For this review, use the dimensioned drawing (mm, ordinates from the lowest corner) and the shaded views. A direction names the side the tool comes from. Coordinates: 2 decimals unless noted, no trailing zeros. Loops run counter-clockwise (first coordinate to the right, second up) from the corner with the lowest first, then second, coordinate; pieces in that order, holes last. Notation, with made-up numbers: M -22.75,27.5 L 34.25,27.5 A23 cw 34.25,47.5 Z; hole C -10.5,-32 d10. An arc over 180 degrees is marked long. One line per item, written item: value.
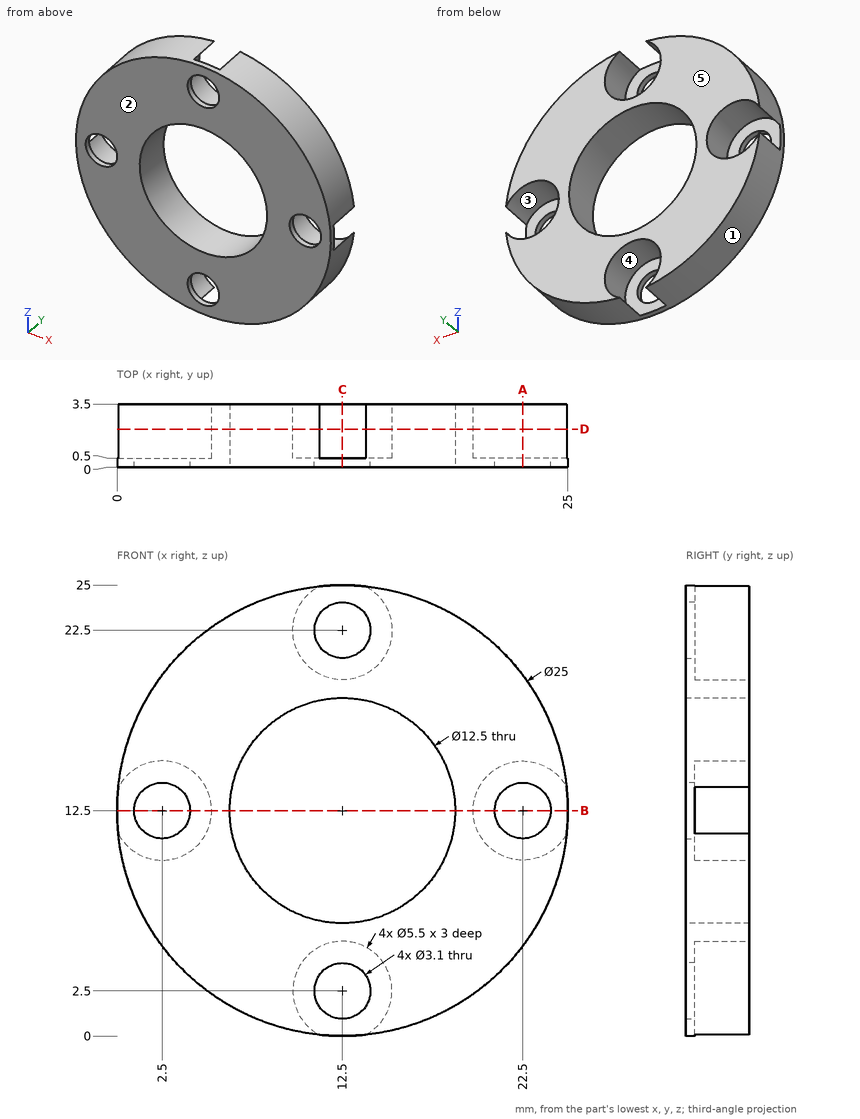
(1) Tool access review of the marked faces 4 and 5: name each direction out of +Z, -Z, +X, -X, +Y, -Y from which nothing blocks a thin tool from reaching the whole face with its end or side.
Reply:
face 4: +Y
face 5: +Z, -Z, +X, -X, +Y
(2) Mouldability with a two-part tool opening along Z and no side actions: class the marked faces 1, 2 and 3 as released by +Z, released by -Z, zero draft, split by the parting line, or undercut.
Reply:
face 1: split by the parting line
face 2: zero draft
face 3: undercut
(3) We need section C-C on x = 12.5. State the section outline as (y, z) points.
Reply:
outline: M 0,0 L 0.5,0 L 0.5,0.95 L 0,0.95 Z; M 0,4.05 L 0.5,4.05 L 0.5,5.25 L 3.5,5.25 L 3.5,6.25 L 0,6.25 Z; M 0,18.75 L 3.5,18.75 L 3.5,19.75 L 0.5,19.75 L 0.5,20.95 L 0,20.95 Z; M 0,24.05 L 0.5,24.05 L 0.5,25 L 0,25 Z
(4) We need section B-B on z = 12.5. State the section outline as (x, y) points.
Reply:
outline: M 0,0 L 0.95,0 L 0.95,0.5 L 0,0.5 Z; M 4.05,0 L 6.25,0 L 6.25,3.5 L 5.25,3.5 L 5.25,0.5 L 4.05,0.5 Z; M 18.75,0 L 20.95,0 L 20.95,0.5 L 19.75,0.5 L 19.75,3.5 L 18.75,3.5 Z; M 24.05,0 L 25,0 L 25,0.5 L 24.05,0.5 Z
(5) We need section A-A on x = 22.5. State the section outline as (y, z) points, then the cut area to 4 significant figures.
Reply:
outline: M 0,5 L 3.5,5 L 3.5,9.75 L 0.5,9.75 L 0.5,10.95 L 0,10.95 Z; M 0,14.05 L 0.5,14.05 L 0.5,15.25 L 3.5,15.25 L 3.5,20 L 0,20 Z
area: 34.45 mm2
(6) To check wall thickness, follow line 1 along Z through (x, y) = (14.25, 2.7); line 2 along X through (y, z) = (3, 10.5); line 3 along X through (y, z) = (1.4, 16.25). State the ranges of each line that lie inside material, in increasing order. Write a range as [from, to].
Reply:
line 1: z = [0.12, 0.38], [4.62, 6.5], [18.5, 20.38], [24.62, 24.88]
line 2: x = [0.16, 0.61], [4.39, 6.58], [18.42, 20.61], [24.39, 24.84]
line 3: x = [0.58, 7.5], [17.5, 24.42]
(7) Insertion check: pin 1 (4.5 mm diameter, centred on x = 12.5, z = 2.5, fed in from -Y); pin 2 (1.6 mm diameter, centred on x = 1.5, z = 12, fed in from +Y); pin 3 (1.5 mm diameter, centred on y = 2.5, z = 17, fed in from -X); pin 4 (2 mm diameter, centred on x = 17, y = 1.5, fed in from +Z). Each pin has a flat end and moves straight along its axis. Give the tip position at first contact, or say it passes through.
Reply:
pin 1: stops at y = 0
pin 2: stops at y = 0.5
pin 3: stops at x = 0.58
pin 4: stops at z = 24.5
(8) We need section D-D on y = 2.1. State the section outline as (x, z) points, then the cut area to 3 significant figures.
Reply:
outline: M 0.07,11.22 A12.5 ccw 11.22,0.07 A2.75 cw long 13.78,0.07 A12.5 ccw 24.93,11.22 A2.75 cw long 24.93,13.78 A12.5 ccw 13.78,24.93 A2.75 cw long 11.22,24.93 A12.5 ccw 0.07,13.78 A2.75 cw long Z; hole C 12.5,12.5 d12.5
area: 275 mm2
